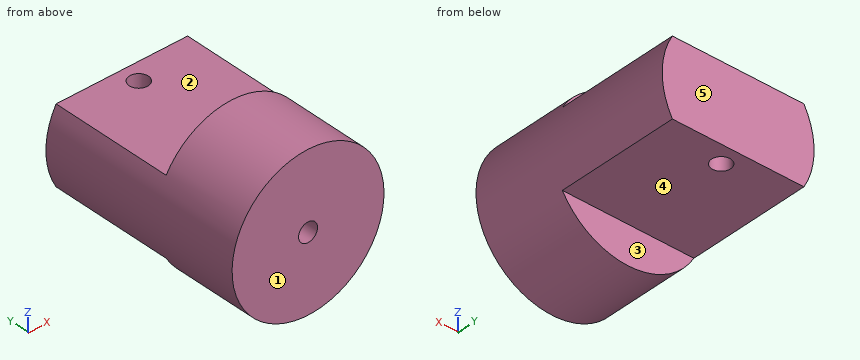
from build123d import *

# Parameters (mm, degrees)
SKETCH1_R           = 50.8
BOSS_EXTRUDE1_DEPTH = 139.7
CUT_EXTRUDE1_START  = 25.4
SKETCH2_W           = 101.6
SKETCH2_H           = 165.1
CUT_EXTRUDE1_DEPTH  = 50.8
CUT_EXTRUDE2_START  = -25.4
SKETCH2_2_W         = 101.6
SKETCH2_2_H         = 165.1
CUT_EXTRUDE2_DEPTH  = 50.8
SKETCH3_R           = 6.35
CUT_EXTRUDE3_DEPTH  = 25.4
SKETCH4_R           = 6.35
CUT_EXTRUDE4_DEPTH  = 168.042419762


with BuildPart() as part:
    # Sketch1 → Boss-Extrude1 (new body)
    with BuildSketch(Plane(origin=(0, 0, 0), x_dir=(1, 0, 0), z_dir=(0, 1, 0))):
        with Locations(Location((0, 0, 0), (0, 0, 270))):
            Circle(SKETCH1_R)
    extrude(amount=BOSS_EXTRUDE1_DEPTH)

    # Sketch2 → Cut-Extrude1 (cut)
    with BuildSketch(Plane.XY.offset(CUT_EXTRUDE1_START)):
        with Locations((0, 139.7)):
            Rectangle(SKETCH2_W, SKETCH2_H)
    extrude(amount=CUT_EXTRUDE1_DEPTH, mode=Mode.SUBTRACT)

    # Sketch2_2 → Cut-Extrude2 (cut)
    with BuildSketch(Plane.XY.offset(CUT_EXTRUDE2_START)):
        with Locations((0, 139.7)):
            Rectangle(SKETCH2_2_W, SKETCH2_2_H)
    extrude(amount=-CUT_EXTRUDE2_DEPTH, mode=Mode.SUBTRACT)

    # Sketch3 → Cut-Extrude3 (cut)
    with BuildSketch(Plane.XZ):
        with Locations(Location((0, 0, 0), (0, 0, 270))):
            Circle(SKETCH3_R)
    extrude(amount=-CUT_EXTRUDE3_DEPTH, mode=Mode.SUBTRACT)

    # Sketch4 → Cut-Extrude4 (cut, through all)
    with BuildSketch(Plane.XY.offset(25.4)):
        with Locations((0, 127)):
            Circle(SKETCH4_R)
    extrude(amount=-CUT_EXTRUDE4_DEPTH, mode=Mode.SUBTRACT)


solid = part.part
Source: CAD feature listing. Evaluate the final solid. Frame: model axes, mm. Face numbers are marked on the shaded views. A direction names the side the tool comes from. Round coordinates to 2 decimals unless told otherwise and drop trailing zeros. Loops run counter-clockwise (first coordinate to the right, second up) from the corner with the lowest first, then second, coordinate; pieces in that order, holes last.
Q1. Section C-C, the plane y = 127. Return loops of the section in (x, z), plus the area to 3 significant figures.
Q2. Access query for the marked faces 4 and 5. Directions: +Z, -Z, +X, -X, +Y, -Y. A direction counts if a zero-diameter tool reaches every point of the face in a straight line with its end or side. Return the directions, or none.
Q3. Section A-A, the plane x = 0. Return loops of the section in (y, z).
Q4. Section D-D, the plane x = -18.5. Return loops of the section in (y, z).
Q5. Section B-B, the plane z = 0. Return loops of the section in (x, y).
Q6. First-contact query: P1, Ø5, axis at y = 27, z = -1, coming from the +X side; P2, Ø10, axis at x = 0, y = 79.5, coming from the -Z side; P3, Ø1, axis at x = -12.5, y = 104.5, coming from the +Z side. Flat tips, straight axial feed; report the tip coordinate or a pass-through.
Q7. Ray query, line 1 (X direction, y = 19, z = 0); line 2 (Z direction, x = 8, y = 87); line 3 (Y direction, x = 27, z = -35). Return the intervals inside material, ascending.
Q8. Mould query, pull axis Y, two halves, no side actions, for the marked faces 1, 2 and 3. Classes: pulls with the +Y half, pulls with the -Y half, needs draft (parallel to the pull), parting line crosses it, or undercut.
Solutions:
1. outline: (-43.99, -25.4) - (-6.35, -25.4) - (-6.35, 25.4) - (-43.99, 25.4) arc R50.8 ccw to start; (6.35, -25.4) - (43.99, -25.4) arc R50.8 ccw to (43.99, 25.4) - (6.35, 25.4) - close
1. area: 4,290 mm2
2. face 4: -Z, +X, -X, +Y
2. face 5: +Z, -Z, +X, -X, +Y
3. outline: (0, -50.8) - (57.15, -50.8) - (57.15, -25.4) - (120.65, -25.4) - (120.65, 25.4) - (57.15, 25.4) - (57.15, 50.8) - (0, 50.8) - (0, 6.35) - (25.4, 6.35) - (25.4, -6.35) - (0, -6.35) - close; (133.35, -25.4) - (139.7, -25.4) - (139.7, 25.4) - (133.35, 25.4) - close
4. outline: (0, -47.31) - (57.15, -47.31) - (57.15, -25.4) - (139.7, -25.4) - (139.7, 25.4) - (57.15, 25.4) - (57.15, 47.31) - (0, 47.31) - close
5. outline: (-50.8, 0) - (-6.35, 0) - (-6.35, 25.4) - (6.35, 25.4) - (6.35, 0) - (50.8, 0) - (50.8, 139.7) - (-50.8, 139.7) - close; hole circle Ø12.7 at (0, 127)
6. P1: stops at x = 50.8
6. P2: stops at z = -25.4
6. P3: stops at z = 25.4
7. line 1: x = -50.8 to -6.35, 6.35 to 50.8
7. line 2: z = -25.4 to 25.4
7. line 3: y = 0 to 57.15
8. face 1: pulls with the -Y half
8. face 2: needs draft
8. face 3: pulls with the +Y half
